For this review, take the finished solid that the model builds, in its own axes (mm). A direction names the side the tool comes from. Round coordinates to 2 decimals unless told otherwise and drop trailing zeros. Order: outer loops, then holes, each group sorted by start corner. A loop starts at its lowest first (then second) coordinate and runs counter-clockwise, first axis right, second up. Notation, with made-up numbers: (86.25, 40) -> (116.25, 40) arc R31 ccw to (116.25, 65) -> close; hole circle Ø1 at (1, 71.25). An arc over 180 degrees is marked (long way). Put each result on its own line as item: value. Start each with the question number.
```python
from build123d import *

# Parameters (mm, degrees)
F0_R     = 6.35
F0_R_2   = 14.351
F1_DEPTH = 17.78
F2_DEPTH = 33.02
F4_DEPTH = 16.002
F5_DEPTH = 16.0782
F6_DEPTH = 16.002
F7_DEPTH = 16.002
F8_R     = 11.176
F8_R_2   = 6.35
F9_DEPTH = 6.35


with BuildPart() as f1:
    # F0 (on Top) → F1 (new body)
    with BuildSketch(Plane.XY):
        with BuildLine():
            Line((44.45, 50.8), (0, 50.8))
            ThreePointArc((0, 50.8), (-25.4, 25.4), (0, 0))
            Line((0, 0), (44.45, 0))
            ThreePointArc((44.45, 0), (19.05, 25.4), (44.45, 50.8))
        make_face()
        with Locations((0, 25.4)):
            Circle(F0_R, mode=Mode.SUBTRACT)
        with BuildLine():
            Line((88.9, 50.8), (44.45, 50.8))
            ThreePointArc((44.45, 50.8), (62.4105122421, 43.3605122421), (69.85, 25.4))
            ThreePointArc((69.85, 25.4), (62.4105122421, 7.4394877579), (44.45, 0))
            Line((44.45, 0), (88.9, 0))
            ThreePointArc((88.9, 0), (114.3, 25.4), (88.9, 50.8))
        make_face()
        with Locations((88.9, 25.4)):
            Circle(F0_R, mode=Mode.SUBTRACT)
        with BuildLine():
            ThreePointArc((69.85, 25.4), (62.4105122421, 43.3605122421), (44.45, 50.8))
            ThreePointArc((44.45, 50.8), (19.05, 25.4), (44.45, 0))
            ThreePointArc((44.45, 0), (62.4105122421, 7.4394877579), (69.85, 25.4))
        make_face()
        with Locations((44.45, 25.4)):
            Circle(F0_R_2, mode=Mode.SUBTRACT)
    extrude(amount=-F1_DEPTH)

    # F0 (on Top) → F2 (join)
    with BuildSketch(Plane.XY):
        with BuildLine():
            ThreePointArc((69.85, 25.4), (62.4105122421, 43.3605122421), (44.45, 50.8))
            ThreePointArc((44.45, 50.8), (19.05, 25.4), (44.45, 0))
            ThreePointArc((44.45, 0), (62.4105122421, 7.4394877579), (69.85, 25.4))
        make_face()
        with Locations((44.45, 25.4)):
            Circle(F0_R_2, mode=Mode.SUBTRACT)
    extrude(amount=F2_DEPTH)

    # F3 (on face) → F4 (cut)
    with BuildSketch(Plane.XY.offset(33.02)):
        with BuildLine():
            ThreePointArc((58.801, 25.4), (58.4694202402, 22.3329073818), (57.4900032571, 19.4075450727))
            Line((57.4900032571, 19.4075450727), (69.1329998976, 19.4075450727))
            ThreePointArc((69.1329998976, 19.4075450727), (69.6701129795, 22.3824014017), (69.85, 25.4))
            ThreePointArc((69.85, 25.4), (69.6236690394, 28.7832509657), (68.9487096774, 32.1062078809))
            Line((68.9487096774, 32.1062078809), (57.1377096774, 32.1062078809))
            ThreePointArc((57.1377096774, 32.1062078809), (58.3789720113, 28.8546982082), (58.801, 25.4))
        make_face()
    extrude(amount=-F4_DEPTH, mode=Mode.SUBTRACT)

    # F3 (on face) → F5 (cut)
    with BuildSketch(Plane.XY.offset(33.02)):
        with BuildLine():
            ThreePointArc((51.1562078809, 12.7122903226), (44.8479805413, 11.0545194403), (38.4575450727, 12.3599967429))
            Line((38.4575450727, 12.3599967429), (38.4575450727, 0.7170001024))
            ThreePointArc((38.4575450727, 0.7170001024), (44.8185804404, 0.0026743837), (51.1562078809, 0.9012903226))
            Line((51.1562078809, 0.9012903226), (51.1562078809, 12.7122903226))
        make_face()
    extrude(amount=-F5_DEPTH, mode=Mode.SUBTRACT)

    # F3 (on face) → F6 (cut)
    with BuildSketch(Plane.XY.offset(33.02)):
        with BuildLine():
            Line((19.7670001024, 19.4075450727), (31.4099967429, 19.4075450727))
            ThreePointArc((31.4099967429, 19.4075450727), (30.1045194403, 25.7979805413), (31.7622903226, 32.1062078809))
            Line((31.7622903226, 32.1062078809), (19.9512903226, 32.1062078809))
            ThreePointArc((19.9512903226, 32.1062078809), (19.0526743837, 25.7685804404), (19.7670001024, 19.4075450727))
        make_face()
    extrude(amount=-F6_DEPTH, mode=Mode.SUBTRACT)

    # F3 (on face) → F7 (cut)
    with BuildSketch(Plane.XY.offset(33.02)):
        with BuildLine():
            Line((38.4575450727, 50.0829998976), (38.4575450727, 38.4400032571))
            ThreePointArc((38.4575450727, 38.4400032571), (44.8479805413, 39.7454805597), (51.1562078809, 38.0877096774))
            Line((51.1562078809, 38.0877096774), (51.1562078809, 49.8987096774))
            ThreePointArc((51.1562078809, 49.8987096774), (44.8185804404, 50.7973256163), (38.4575450727, 50.0829998976))
        make_face()
    extrude(amount=-F7_DEPTH, mode=Mode.SUBTRACT)

    # F8 (on Top) → F9 (cut)
    with BuildSketch(Plane.XY):
        with Locations((0, 25.4)):
            Circle(F8_R)
        with Locations((0, 25.4)):
            Circle(F8_R_2, mode=Mode.SUBTRACT)
        with Locations((88.9, 25.4)):
            Circle(F8_R)
        with Locations((88.9, 25.4)):
            Circle(F8_R_2, mode=Mode.SUBTRACT)
    extrude(amount=-F9_DEPTH, mode=Mode.SUBTRACT)


solid = f1.part
```
Item 1: Consider section D-D, the plane x = 80. Write out the cut boundary in (y, z).
Item 2: Consider section B-B, the plane z = -11.5. Write out the cut boundary in (x, y).
Item 3: Mouldability with a two-part tool opening along X and no side actions: class faces 4 (the face through (114.294, 24.841, -8.766)), 5 (the face through (25, 26, 17.018)), 6 (the face through (2.93, 19.766, -11.985)) as +X half, -X half, draft (parallel to the pull), parting line (faces both ways), or undercut.
Item 4: Consider section C-C, the plane y = 44. Write out the cut boundary in (x, z).
Item 5: For L1, parallel to X at y = 26, z = -2; L2, parallel to Y at x = 88.9, z = -10; L3, parallel to X at y = 20, z = -5.5, list the stretches that pass through material, from the lowest coordinate up.
Item 6: Consider section A-A, the plane x = 5. Write out the cut boundary in (y, z).
Item 7: Tool access review of faces 1 (the face through (26, 19.408, 25)), 2 (the face through (45, 45, 17.018)), 3 (the face through (94, 21, -6.35)): name each direction out of +Z, -Z, +X, -X, +Y, -Y from which nothing blocks a thin tool from reaching the whole face with its end or side.
Item 8: Insertion check: pin 1 Ø3.5 at (y, z) = (43, 22) entering from -X; pin 2 Ø4 at (x, y) = (12, 36) entering from +Z; pin 3 Ø9.5 at (y, z) = (7.5, 27.5) entering from -X; pin 4 Ø14 at (x, y) = (47.5, 6) entering from +Z. Each pin has a flat end and moves straight along its axis. Give the tip position at first contact, or say it passes through.
Evaluation:
1. outline: (0, -17.78) -> (50.8, -17.78) -> (50.8, 0) -> (32.16, 0) -> (32.16, -6.35) -> (18.64, -6.35) -> (18.64, 0) -> (0, 0) -> close
2. outline: (0, 0) -> (88.9, 0) arc R25.4 ccw to (88.9, 50.8) -> (0, 50.8) arc R25.4 ccw to start; hole circle Ø12.7 at (0, 25.4); hole circle Ø28.7 at (44.45, 25.4); hole circle Ø12.7 at (88.9, 25.4)
3. face 4: +X half
3. face 5: draft
3. face 6: undercut
4. outline: (-17.3, -17.78) -> (106.2, -17.78) -> (106.2, 0) -> (61.75, 0) -> (61.75, 33.02) -> (51.16, 33.02) -> (51.16, 17.02) -> (38.46, 17.02) -> (38.46, 33.02) -> (27.15, 33.02) -> (27.15, 0) -> (-17.3, 0) -> close
5. L1: x = -25.39 to -11.16, 11.16 to 30.11, 58.79 to 77.74, 100.06 to 114.29
5. L2: y = 0 to 19.05, 31.75 to 50.8
5. L3: x = -24.82 to -9.78, 9.78 to 31.15, 57.75 to 79.12, 98.68 to 113.72
6. outline: (0, -17.78) -> (21.49, -17.78) -> (21.49, -6.35) -> (15.4, -6.35) -> (15.4, 0) -> (0, 0) -> close; (29.31, -17.78) -> (50.8, -17.78) -> (50.8, 0) -> (35.4, 0) -> (35.4, -6.35) -> (29.31, -6.35) -> close
7. face 1: +Z, +X, -X
7. face 2: +Z, +Y, -Y
7. face 3: +Z
8. pin 1: stops at x = 24.6
8. pin 2: stops at z = 0
8. pin 3: stops at x = 22.72
8. pin 4: stops at z = 33.02
